Input: part model. Units: mm. Frame: model coordinates. A direction names the side the tool comes from. Round coordinates to 2 decimals unless told otherwise and drop trailing zeros. Loops run counter-clockwise (first coordinate to the right, second up) from the corner with the lowest first, then second, coordinate; pieces in that order, holes last.
1) Section C-C, the plane z = -8.5. Return loops of the section in (x, y).
2) Section B-B, the plane y = 12. Return loops of the section in (x, z), and give its area (3 significant figures).
3) Draft query along Z for faces 1 (the face through (9.9, 9.9, -20)), 2 (the face through (3, 10, -10)), 3 (the face through (12, 2, -2)), 4 (the face through (8.3, 2.4, -6.1)). Return one class per face: pulls with the +Z half, pulls with the -Z half, needs draft (parallel to the pull), parting line crosses it, or undercut.
4) Section A-A, the plane x = 11.5. Return loops of the section in (y, z).
5) First-contact query: pin 1 (4 mm diameter, centred on x = 11, z = -8, fed in from +Y); pin 2 (2 mm diameter, centred on x = 18, y = 10.5, fed in from +Z); pin 3 (2 mm diameter, centred on x = 7.5, z = -8.5, fed in from +Y); pin 4 (3 mm diameter, centred on x = 11.5, z = -8.5, fed in from -Y). Flat tips, straight axial feed; report the tip coordinate or a pass-through.
6) Ray query, line 1 along X through (y, z) = (1.25, -8.5); line 2 along Y through (x, z) = (4.75, -3.25); line 3 along Z through (x, y) = (6, 16.5). Return the intervals inside material, ascending.
7) Access query for faces 5 (the face through (12, 3, -13)), 6 (the face through (9.9, 0, -10.1)), 7 (the face through (13.2, 1.8, -6.8)). Directions: +Z, -Z, +X, -X, +Y, -Y. A direction counts if a zero-diameter tool reaches every point of the face in a straight line with its end or side. Return the directions, or none.
8) Section D-D, the plane x = 6. Return loops of the section in (y, z), and give its area (3 significant figures).
from build123d import *

# Parameters (mm, degrees)
IZIM1_W                     = 20
IZIM1_H                     = 20
Y_KSEKLIK_EKSTR_ZYON1_DEPTH = 20
KES_EKSTR_ZYON1_DEPTH       = 17
IZIM3_W                     = 17.326301073
IZIM3_H                     = 17.919650739
KES_EKSTR_ZYON2_DEPTH       = 17
IZIM6_R                     = 2
KES_EKSTR_ZYON3_DEPTH       = 17
IZIM7_R                     = 2
KES_EKSTR_ZYON4_DEPTH       = 17
IZIM5_R                     = 2
KES_EKSTR_ZYON5_DEPTH       = 17
IZIM8_R                     = 4
KES_EKSTR_ZYON6_DEPTH       = 1.2


with BuildPart() as part:
    # Çizim1 → Yükseklik-Ekstrüzyon1 (new body)
    with BuildSketch(Plane(origin=(0, 0, 0), x_dir=(1, 0, 0), z_dir=(0, 1, 0))):
        with Locations((10, 10)):
            Rectangle(IZIM1_W, IZIM1_H)
    extrude(amount=Y_KSEKLIK_EKSTR_ZYON1_DEPTH)

    # Çizim2 → Kes-Ekstrüzyon1 (cut)
    with BuildSketch(Plane(origin=(20, 0, 0), x_dir=(0, 0, -1), z_dir=(1, 0, 0))):
        Polygon((20, 20), (0, 0), (0, 20), align=None)
    extrude(amount=-KES_EKSTR_ZYON1_DEPTH, mode=Mode.SUBTRACT)

    # Çizim3 → Kes-Ekstrüzyon2 (cut)
    with BuildSketch(Plane(origin=(20, 0, 0), x_dir=(0, 0, -1), z_dir=(1, 0, 0))):
        with Locations((8.336849464, 11.95982537)):
            Rectangle(IZIM3_W, IZIM3_H)
    extrude(amount=-KES_EKSTR_ZYON2_DEPTH, mode=Mode.SUBTRACT)

    # Çizim6 → Kes-Ekstrüzyon3 (cut)
    with BuildSketch(Plane(origin=(3, 0, 0), x_dir=(0, 0, -1), z_dir=(1, 0, 0))):
        with Locations((7.5, 12.5)):
            Circle(IZIM6_R)
    extrude(amount=-KES_EKSTR_ZYON3_DEPTH, mode=Mode.SUBTRACT)

    # Çizim7 → Kes-Ekstrüzyon4 (cut)
    with BuildSketch(Plane.XY.offset(-17)):
        with Locations((11.5, 11.5)):
            Circle(IZIM7_R)
    extrude(amount=-KES_EKSTR_ZYON4_DEPTH, mode=Mode.SUBTRACT)

    # Çizim5 → Kes-Ekstrüzyon5 (cut)
    with BuildSketch(Plane(origin=(0, 3, 0), x_dir=(1, 0, 0), z_dir=(0, 1, 0))):
        with Locations((11.5, 8.5)):
            Circle(IZIM5_R)
    extrude(amount=-KES_EKSTR_ZYON5_DEPTH, mode=Mode.SUBTRACT)

    # Çizim8 → Kes-Ekstrüzyon6 (cut)
    with BuildSketch(Plane(origin=(0, 3, 0), x_dir=(1, 0, 0), z_dir=(0, 1, 0))):
        with Locations((11.5, 8.5)):
            Circle(IZIM8_R)
    extrude(amount=-KES_EKSTR_ZYON6_DEPTH, mode=Mode.SUBTRACT)


solid = part.part
Final values:
1. outline: (0, 0) - (9.5, 0) - (9.5, 1.8) - (7.5, 1.8) - (7.5, 3) - (3, 3) - (3, 10.77) - (0, 10.77) - close; (0, 14.23) - (3, 14.23) - (3, 20) - (0, 20) - close; (13.5, 0) - (20, 0) - (20, 3) - (15.5, 3) - (15.5, 1.8) - (13.5, 1.8) - close
2. outline: (0, -20) - (9.56, -20) - (9.56, -17) - (3, -17) - (3, -9.44) - (0, -9.44) - close; (0, -5.56) - (3, -5.56) - (3, 0) - (0, 0) - close; (13.44, -20) - (20, -20) - (20, -17) - (13.44, -17) - close
2. area: 87.8 mm2
3. face 1: pulls with the -Z half
3. face 2: needs draft
3. face 3: pulls with the +Z half
3. face 4: undercut
4. outline: (0, -20) - (9.5, -20) - (9.5, -17) - (3, -17) - (3, -12.5) - (1.8, -12.5) - (1.8, -10.5) - (0, -10.5) - close; (0, -6.5) - (1.8, -6.5) - (1.8, -4.5) - (3, -4.5) - (3, -3) - (0, 0) - close; (13.5, -20) - (20, -20) - (17, -17) - (13.5, -17) - close
5. pin 1: stops at y = 1.8
5. pin 2: stops at z = -17
5. pin 3: stops at y = 3
5. pin 4: passes through
6. line 1: x = 0 to 9.5, 13.5 to 20
6. line 2: y = 0 to 3
6. line 3: z = -20 to -17
7. face 5: +Z, +X, +Y
7. face 6: +Z, -Z, +X, -X, -Y
7. face 7: +Y
8. outline: (0, -20) - (20, -20) - (17, -17) - (3, -17) - (3, -3) - (0, 0) - close
8. area: 102 mm2
